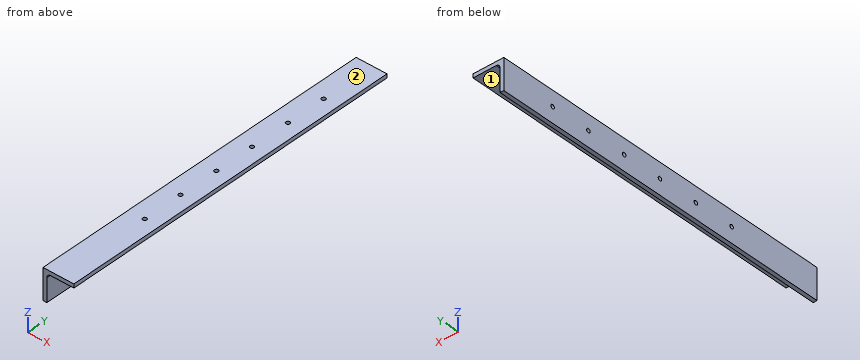
from build123d import *

# Parameters (mm, degrees)
BOSS_EXTRUDE1_DEPTH      = 577.85
FILLET1_R                = 6.35
F_0_257_DIAMETER_HOLE1_D = 6.5278
LPATTERN1_COUNT          = 6
LPATTERN1_PITCH          = 66.04
F_0_257_DIAMETER_HOLE2_D = 6.5278
LPATTERN2_COUNT          = 6
LPATTERN2_PITCH          = 66.04


with BuildPart() as part:
    # Sketch2 → Boss-Extrude1 (new body)
    with BuildSketch(Plane(origin=(0, 6.35, 0), x_dir=(1, 0, 0), z_dir=(0, 1, 0))):
        Polygon((-304.8, -406.4), (-304.8, -457.2), (-254, -457.2), (-254, -450.85), (-298.45, -450.85), (-298.45, -406.4), align=None)
    extrude(amount=BOSS_EXTRUDE1_DEPTH)

    # Fillet1
    fillet1_edges = [part.edges().sort_by_distance(p)[0] for p in [
        (-298.45, 295.275, 450.85),
    ]]
    fillet(fillet1_edges, radius=FILLET1_R)

    # F (0.257) Diameter Hole1 (through all)
    with Locations(Plane.XY.offset(457.2)):
        with Locations((-535.515028223, 347.01452534), (-277.982504407, 164.015269696)):
            f_0_257_diameter_hole1 = Hole(F_0_257_DIAMETER_HOLE1_D / 2)

    # LPattern1: F (0.257) Diameter Hole1 ×6
    with Locations(*[(0, i * LPATTERN1_PITCH, 0) for i in range(1, LPATTERN1_COUNT)]):
        add(f_0_257_diameter_hole1, mode=Mode.SUBTRACT)

    # F (0.257) Diameter Hole2 (through all)
    with Locations(Plane.ZY.offset(304.8)):
        with Locations((431.8, 164.015269696)):
            f_0_257_diameter_hole2 = Hole(F_0_257_DIAMETER_HOLE2_D / 2)

    # LPattern2: F (0.257) Diameter Hole2 ×6
    with Locations(*[(0, i * LPATTERN2_PITCH, 0) for i in range(1, LPATTERN2_COUNT)]):
        add(f_0_257_diameter_hole2, mode=Mode.SUBTRACT)


solid = part.part
The model under review builds one solid part; all positions refer to its coordinate system, in mm. Face numbers are marked on the shaded views. A direction names the side the tool comes from. Coordinates: 2 decimals unless noted, no trailing zeros. Loops run counter-clockwise (first coordinate to the right, second up) from the corner with the lowest first, then second, coordinate; pieces in that order, holes last. Notation, with made-up numbers: (29, -33) -> (47, -33) arc R17 ccw to (47, -1) -> close; hole circle Ø4 at (-19.75, 43). An arc over 180 degrees is marked (long way). Use a Markdown table: item, result. Add a question column.
1. Add section C-C on z = 415. Write out the cut boundary in (x, y), plus the area to 3 significant figures.
2. Add section A-A on y = 439. Write out the cut boundary in (x, z), plus the area to 3 significant figures.
3. Add section B-B on x = -270. Write out the cut boundary in (y, z), plus the area to 3 significant figures.
4. Machinability: for the marked faces 1 and 2, which of the approach directions +Z, -Z, +X, -X, +Y, -Y give a long, thin tool a straight path to every point of the face, cutting with its end or side? Answer none if there is none.
5. To check wall thickness, follow line 1 (Z direction, x = -271, y = 552); line 2 (X direction, y = 64, z = 426). State the ranges of each line that lie inside material, in increasing order.
6. Clearance check with flat-ended pins moving along their axes: pin 1 Ø8.5 at (x, y) = (-277.98, 296.1) entering from -Z; pin 2 Ø6 at (y, z) = (492, 443.5) entering from +X; pin 3 Ø19 at (y, z) = (347.5, 422.5) entering from +X. State where each tip first meets the part, or that it passes through.
Returned:
| question | item | result |
|---|---|---|
| 1 | outline | (-304.8, 6.35) -> (-298.45, 6.35) -> (-298.45, 584.2) -> (-304.8, 584.2) -> close |
| 1 | area | 3,670 mm² |
| 2 | outline | (-304.8, 406.4) -> (-298.45, 406.4) -> (-298.45, 444.5) arc R6.35 cw to (-292.1, 450.85) -> (-254, 450.85) -> (-254, 457.2) -> (-304.8, 457.2) -> close |
| 2 | area | 613 mm² |
| 3 | outline | (6.35, 450.85) -> (584.2, 450.85) -> (584.2, 457.2) -> (6.35, 457.2) -> close |
| 3 | area | 3,670 mm² |
| 4 | face 1 | -Z, +X, +Y, -Y |
| 4 | face 2 | +Z, +X, -X, +Y, -Y |
| 5 | line 1 | z = 450.85 to 457.2 |
| 5 | line 2 | x = -304.8 to -298.45 |
| 6 | pin 1 | stops at z = 450.85 |
| 6 | pin 2 | stops at x = -298.13 |
| 6 | pin 3 | stops at x = -298.45 |
